The model under review builds one solid part; all positions refer to its coordinate system, in mm. A direction names the side the tool comes from. Round coordinates to 2 decimals unless told otherwise and drop trailing zeros. Loops run counter-clockwise (first coordinate to the right, second up) from the corner with the lowest first, then second, coordinate; pieces in that order, holes last. Notation, with made-up numbers: (8, -28.75) -> (24, -28.75) arc R28 ccw to (24, 9.25) -> close; hole circle Ø7 at (44.5, 86.25). An arc over 180 degrees is marked (long way). Use a Markdown table: item, result. Add a question column.
1) Wall thickness on probe 1 along Y at (x, z) = (2.5, 19.5); probe 2 along Y at (x, z) = (0.95, -128); probe 3 along Z at (x, y) = (0.55, -63.5): over which ranges is each line inside the solid? List them lowest first.
2) Consider section B-B on x = 0.75. State how many separate pieces and enclosed holes the cut face has, plus the area to 3 significant figures.
3) Consider section A-A on z = -197. Give the boundary of the cut face in (x, y), plus the area to 3 significant figures.
4) For faces 1 (the flat face through (1.479, -105.15, 126.445)), 2 (the cylindrical face through (1.479, 62.081, 76.516)), list the 3-axis set-ups (+Z, -Z, +X, -X, +Y, -Y) from which the entire face can be reached by the end or side of a thin tool; tool diameter is ignored.
5) Mouldability with a two-part tool opening along Z and no side actions: class faces 3 (the cylindrical face through (1.479, -142.463, -185.668)), 4 (the flat face through (0, -28, -52)), 5 (the cylindrical face through (1.479, 54.364, -198.037)) as released by +Z, released by -Z, zero draft, split by the parting line, or undercut.
from build123d import *

# Parameters (mm, degrees)
BOSS_EXTRUDE1_DEPTH = 3


with BuildPart() as part:
    # Sketch3 → Boss-Extrude1 (new body)
    with BuildSketch(Plane(origin=(0, 0, 0), x_dir=(0, 0, -1), z_dir=(1, 0, 0))):
        with BuildLine():
            Line((296.275579055, -106.762485274), (296.275579055, 28.183515817))
            ThreePointArc((296.275579055, 28.183515817), (291.290828585, 43.295682658), (278.29309192, 52.476323454))
            ThreePointArc((278.29309192, 52.476323454), (59.883707169, 97.109052306), (-163.023302782, 99.793218303))
            ThreePointArc((-163.023302782, 99.793218303), (-179.612272596, 91.682532966), (-186.324420945, 74.480085446))
            Line((-186.324420945, 74.480085446), (-186.324420945, -37.496742321))
            ThreePointArc((-186.324420945, -37.496742321), (-184.257501936, -47.533043008), (-178.393135002, -55.935940492))
            Line((-178.393135002, -55.935940492), (-73.021933987, -155.761288823))
            ThreePointArc((-73.021933987, -155.761288823), (-64.95546345, -160.91780672), (-55.55321993, -162.722090651))
            Line((-55.55321993, -162.722090651), (95.783603989, -162.722090651))
            ThreePointArc((95.783603989, -162.722090651), (99.360261791, -162.469009329), (102.86564516, -161.714808681))
            ThreePointArc((102.86564516, -161.714808681), (186.857264311, -142.254171864), (272.475288326, -132.112059831))
            ThreePointArc((272.475288326, -132.112059831), (289.393038593, -124.148217707), (296.275579055, -106.762485274))
        make_face()
        with BuildLine():
            Line((-140.201640509, -57.128850103), (-87.96769136, -106.613644033))
            ThreePointArc((-87.96769136, -106.613644033), (-81.148094961, -107.861160131), (-77.251705961, -102.126934444))
            ThreePointArc((-77.251705961, -102.126934444), (-76.008202248, -79.905919655), (-73.146568748, -57.834878595))
            ThreePointArc((-73.146568748, -57.834878595), (-74.384458899, -52.907294986), (-78.839479519, -50.464705473))
            ThreePointArc((-78.839479519, -50.464705473), (-106.402906269, -47.617091315), (-133.882969985, -44.053736318))
            ThreePointArc((-133.882969985, -44.053736318), (-141.821884271, -48.281517128), (-140.201640509, -57.128850103))
        make_face(mode=Mode.SUBTRACT)
        with BuildLine():
            Line((63.109549173, -54.772090651), (16.875579055, -54.772090651))
            ThreePointArc((16.875579055, -54.772090651), (-3.030152717, -54.586152411), (-22.928937744, -54.02840258))
            ThreePointArc((-22.928937744, -54.02840258), (-26.745457872, -55.128882574), (-29.161505638, -58.281594946))
            ThreePointArc((-29.161505638, -58.281594946), (-39.202655269, -93.85476168), (-44.863942819, -130.381802358))
            ThreePointArc((-44.863942819, -130.381802358), (-43.235628118, -135.248430754), (-38.54143859, -137.322090651))
            Line((-38.54143859, -137.322090651), (68.867981086, -137.322090651))
            ThreePointArc((68.867981086, -137.322090651), (73.52045107, -137.108595997), (78.133815642, -136.469906519))
            ThreePointArc((78.133815642, -136.469906519), (82.01587994, -134.088804485), (83.305445186, -129.72107148))
            ThreePointArc((83.305445186, -129.72107148), (78.315586037, -94.014248859), (69.14438597, -59.146427513))
            ThreePointArc((69.14438597, -59.146427513), (66.836279581, -55.980691964), (63.109549173, -54.772090651))
        make_face(mode=Mode.SUBTRACT)
        with BuildLine():
            Line((124.985022972, -54.772090651), (113.865129032, -54.772090651))
            ThreePointArc((113.865129032, -54.772090651), (108.895908777, -57.16869337), (107.677632388, -62.54946071))
            ThreePointArc((107.677632388, -62.54946071), (112.731044206, -90.235858533), (115.209207632, -118.270342681))
            ThreePointArc((115.209207632, -118.270342681), (117.754129966, -123.091695748), (123.099684529, -124.162733326))
            ThreePointArc((123.099684529, -124.162733326), (146.984385828, -118.546914937), (171.026989965, -113.651043346))
            ThreePointArc((171.026989965, -113.651043346), (175.823137855, -109.575179128), (174.754311259, -103.372493144))
            ThreePointArc((174.754311259, -103.372493144), (152.912685544, -78.94134113), (129.173611289, -56.349436473))
            ThreePointArc((129.173611289, -56.349436473), (127.222895395, -55.179496351), (124.985022972, -54.772090651))
        make_face(mode=Mode.SUBTRACT)
        with BuildLine():
            Line((245.475579055, -54.772090651), (189.600512971, -54.772090651))
            ThreePointArc((189.600512971, -54.772090651), (184.070618685, -58.000749725), (184.164076639, -64.403501933))
            ThreePointArc((184.164076639, -64.403501933), (195.077427987, -83.649499652), (204.927221509, -103.460891158))
            ThreePointArc((204.927221509, -103.460891158), (207.64086464, -106.360834644), (211.546531528, -107.081457582))
            ThreePointArc((211.546531528, -107.081457582), (229.074894441, -104.882673663), (246.646711113, -103.063493647))
            ThreePointArc((246.646711113, -103.063493647), (254.86076358, -98.973792541), (258.175579055, -90.417606976))
            Line((258.175579055, -90.417606976), (258.175579055, -67.472090651))
            ThreePointArc((258.175579055, -67.472090651), (254.455835176, -58.49183453), (245.475579055, -54.772090651))
        make_face(mode=Mode.SUBTRACT)
        with BuildLine():
            ThreePointArc((-63.423694749, 73.386671701), (-61.283949627, 80.468910348), (-67.303330529, 84.770499241))
            ThreePointArc((-67.303330529, 84.770499241), (-101.974198169, 84.203420455), (-136.612578489, 82.599285182))
            ThreePointArc((-136.612578489, 82.599285182), (-153.291167029, 64.166222989), (-135.240146412, 47.0748874))
            ThreePointArc((-135.240146412, 47.0748874), (-114.033668366, 47.33348842), (-92.825838328, 47.431113877))
            ThreePointArc((-92.825838328, 47.431113877), (-90.125310843, 48.036382475), (-87.938719053, 49.732853847))
            ThreePointArc((-87.938719053, 49.732853847), (-76.344200811, 62.246895478), (-63.423694749, 73.386671701))
        make_face(mode=Mode.SUBTRACT)
        with BuildLine():
            ThreePointArc((69.231514749, 75.634749617), (67.555654459, 76.763975447), (65.609872244, 77.309493785))
            ThreePointArc((65.609872244, 77.309493785), (29.88891223, 80.823452233), (-5.923738689, 83.229470179))
            ThreePointArc((-5.923738689, 83.229470179), (-8.378239234, 82.871089318), (-10.508168123, 81.599707119))
            ThreePointArc((-10.508168123, 81.599707119), (-22.236344306, 69.777534825), (-32.604624722, 56.746317095))
            ThreePointArc((-32.604624722, 56.746317095), (-33.101585539, 50.220258497), (-27.57017357, 46.721702724))
            ThreePointArc((-27.57017357, 46.721702724), (28.340185633, 44.900589153), (84.202879174, 41.960488643))
            ThreePointArc((84.202879174, 41.960488643), (90.139619886, 45.193850997), (89.79812833, 51.945362376))
            ThreePointArc((89.79812833, 51.945362376), (80.12600177, 64.320669452), (69.231514749, 75.634749617))
        make_face(mode=Mode.SUBTRACT)
        with BuildLine():
            ThreePointArc((145.858420697, 39.213689288), (147.772723887, 37.715638334), (150.109622506, 37.04659558))
            ThreePointArc((150.109622506, 37.04659558), (203.802057157, 31.881595955), (257.384776304, 25.681033985))
            ThreePointArc((257.384776304, 25.681033985), (264.392806933, 30.68986561), (259.959983781, 38.075728216))
            ThreePointArc((259.959983781, 38.075728216), (197.151625063, 54.570624598), (133.51792631, 67.521451383))
            ThreePointArc((133.51792631, 67.521451383), (126.665438798, 63.936972071), (128.357377735, 56.390951951))
            ThreePointArc((128.357377735, 56.390951951), (137.453954347, 48.154898666), (145.858420697, 39.213689288))
        make_face(mode=Mode.SUBTRACT)
    extrude(amount=BOSS_EXTRUDE1_DEPTH)


solid = part.part
Result set:
| question | item | result |
|---|---|---|
| 1 | probe 1 | -162.72 to -137.32, -54.15 to 46.53, 72.77 to 102.92 |
| 1 | probe 2 | -154.87 to -122.95, -55.53 to 56.71, 65.82 to 87.79 |
| 1 | probe 3 | -296.28 to -257.54, -183.71 to -137.11, -107.9 to -70.53, 30.93 to 74.04, 133.48 to 170.41 |
| 2 | separate pieces | 1 |
| 2 | enclosed holes | 7 |
| 2 | area | 82,700 mm2 |
| 3 | outline | (0, -140.55) -> (3, -140.55) -> (3, -87.31) -> (0, -87.31) -> close; (0, -54.77) -> (3, -54.77) -> (3, 32.59) -> (0, 32.59) -> close; (0, 54.61) -> (3, 54.61) -> (3, 74.16) -> (0, 74.16) -> close |
| 3 | area | 480 mm2 |
| 4 | face 1 | +Z, +X, -X, -Y |
| 4 | face 2 | +X, -X |
| 5 | face 3 | released by -Z |
| 5 | face 4 | zero draft |
| 5 | face 5 | undercut |
